Could you check a few things on this model? Use its own coordinates, in mm. A direction names the side the tool comes from. Coordinates: 2 decimals unless noted, no trailing zeros. Order: outer loops, then holes, each group sorted by start corner. A loop starts at its lowest first (then second) coordinate and runs counter-clockwise, first axis right, second up. Notation, with made-up numbers: (2.25, -37.75) - (32.25, -37.75) arc R31 ccw to (32.25, -4.75) - close; hole circle Ø9 at (-6.5, -25.5). An arc over 180 degrees is marked (long way). One line per item, written item: value.
from build123d import *

# Parameters (mm, degrees)
F2_R     = 70.629531
F3_DEPTH = 152.4
F4_R     = 53.301947
F5_DEPTH = 459.74


with BuildPart() as f1:
    # F0 (on Right) → F1 (revolve)
    with BuildSketch(Plane.YZ):
        Polygon((95.25, 323.85), (0, 323.85), (0, -184.15), (95.25, -184.15), (95.25, -69.85), (149.225, -69.85), (149.225, 0), (95.25, 0), (95.25, 152.4), (149.225, 152.4), (149.225, 222.25), (95.25, 222.25), align=None)
    revolve(axis=Axis((0, 0, 7.681185), (0, 0, -1)))

    # F2 (on face) → F3 (join)
    with BuildSketch(Plane.XY.offset(323.85)):
        Circle(F2_R)
    extrude(amount=F3_DEPTH)

    # F4 (on face) → F5 (join)
    with BuildSketch(Plane(origin=(0, 0, -184.15), x_dir=(1, 0, 0), z_dir=(0, 0, -1))):
        Circle(F4_R)
    extrude(amount=F5_DEPTH)


solid = f1.part
Item 1: I want a section at B-B on x = -120. Please give me the cut outline in (y, z), then the cut area to 3 significant figures.
Conclusion:
outline: (-88.7, -69.85) - (88.7, -69.85) - (88.7, 0) - (-88.7, 0) - close; (-88.7, 152.4) - (88.7, 152.4) - (88.7, 222.25) - (-88.7, 222.25) - close
area: 24,800 mm²
Item 2: I want a section at C-C on y = 0. Please give me the cut outline in (x, z) (3 decimals).
Conclusion:
outline: (-149.225, -69.85) - (-95.25, -69.85) - (-95.25, -184.15) - (-53.302, -184.15) - (-53.302, -643.89) - (53.302, -643.89) - (53.302, -184.15) - (95.25, -184.15) - (95.25, -69.85) - (149.225, -69.85) - (149.225, 0) - (95.25, 0) - (95.25, 152.4) - (149.225, 152.4) - (149.225, 222.25) - (95.25, 222.25) - (95.25, 323.85) - (70.63, 323.85) - (70.63, 476.25) - (-70.63, 476.25) - (-70.63, 323.85) - (-95.25, 323.85) - (-95.25, 222.25) - (-149.225, 222.25) - (-149.225, 152.4) - (-95.25, 152.4) - (-95.25, 0) - (-149.225, 0) - close
Item 3: If I drill on probe 1 along Z at (x, y) = (-69.5, 80.5); probe 2 along Y at (x, z) = (1.5, 238.5); probe 3 along Z at (x, y) = (66.5, 47.5), over which ranges is the centre line in solid material (lowest first)?
Conclusion:
probe 1: -69.85 to 0, 152.4 to 222.25
probe 2: -95.24 to 95.24
probe 3: -184.15 to 323.85
Item 4: I want a section at D-D on z = 199.5. Please give me the cut outline in (x, y) (3 decimals).
Conclusion:
outline: circle Ø298.45 at (0, 0)
Item 5: I want a section at A-A on y = 119. Please give me the cut outline in (x, z), then the cut area to 3 significant figures.
Conclusion:
outline: (-90.04, -69.85) - (90.04, -69.85) - (90.04, 0) - (-90.04, 0) - close; (-90.04, 152.4) - (90.04, 152.4) - (90.04, 222.25) - (-90.04, 222.25) - close
area: 25,200 mm²
Item 6: I'm going to push flat-ended pins straight in: pin 1 Ø1.5 at (x, z) = (-32, 307) entering from +Y; pin 2 Ø2 at (x, z) = (31, 69.5) entering from +Y; pin 3 Ø4 at (x, y) = (112, -72.5) entering from +Z. Where does each tip first touch, or does it pass through?
Conclusion:
pin 1: y = 89.98
pin 2: y = 90.4
pin 3: z = 222.25
Item 7: For faces 1 (the face through (0, -71, 323.85)), 2 (the face through (2, -97, 152.4)), 3 (the face through (-90.8, -118.42, 187.81)), 4 (the face through (-1, 1, 476.25)), 5 (the face through (-6.94, -52.85, -410.8)), which set-ups out of +Z, -Z, +X, -X, +Y, -Y let a thin tool reach every point of the face, with its end or its side?
Conclusion:
face 1: +Z
face 2: none
face 3: +Z, -Z
face 4: +Z, +X, -X, +Y, -Y
face 5: -Z
Item 8: Thinking about a two-plate mould opening in Z: for faces 6 (the face through (-1, -1, -643.89)), 7 (the face through (-57.958, -75.587, 77.267)), 8 (the face through (-57.958, -75.587, -126.2)), which applies, pulls with the +Z half, pulls with the -Z half, needs draft (parallel to the pull), parting line crosses it, or undercut?
Conclusion:
face 6: pulls with the -Z half
face 7: undercut
face 8: needs draft
